Answer from the drawing. Dimensions are ordinates in mm from the lowest x, y and z of the part. Coordinates: 2 decimals unless noted, no trailing zeros. Write each loop counter-clockwise with the first axis right and the second up, starting at its lowest first coordinate (ties: lowest second). Pieces come first, ordered by that corner, then holes. Notation, with made-up numbers: M 63,-11 L 84,-11 A24 cw 84,24 Z; hole C 28.5,87 d7. An arc over 180 degrees is marked long. Put each result on its own line as item: value. Start each with the question number.
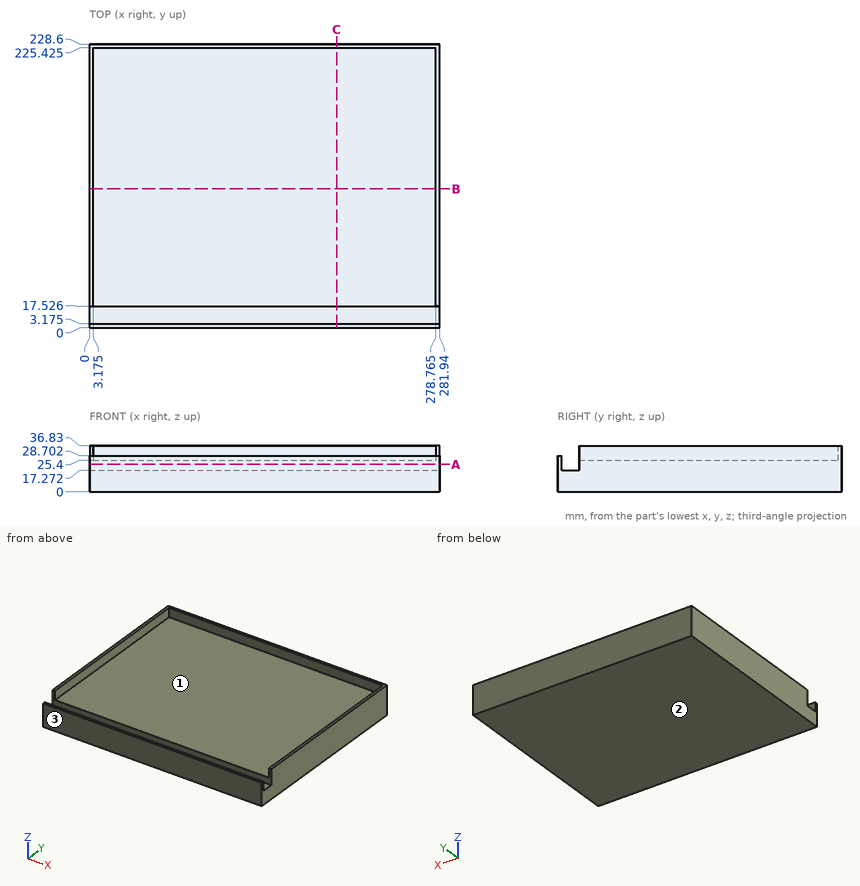
1) A cutting plane is placed at C-C on x = 199. Write down the section's boundary in (y, z) (3 decimals).
2) Determine the mould class of the marked faces 1, 2 and 3 for opening direction Y: +Y half, -Y half, draft (parallel to the pull), parting line (faces both ways), or undercut.
3) Given pin 1 Ø16 at (x, y) = (81.5, 7.5) entering from +Z; pin 2 Ø10 at (x, y) = (57.5, 185.5) entering from +Z; pin 3 Ø3.5 at (x, z) = (150, 33) entering from -Y (3 decimals), each flat-ended and moving along its own axis, determine where each tip first touches the part or whether it passes through.
4) A cutting plane is placed at B-B on y = 112. Write down the section's boundary in (x, z) (3 decimals).
5) Straight lines are drawn through the part: probe 1 along X at (y, z) = (146.5, 27) (3 decimals); probe 2 along Y at (x, z) = (138, 23) (3 decimals); probe 3 along Y at (x, z) = (58, 27) (3 decimals). For each, find the intervals that lie inside material, in ascending order.
6) A cutting plane is placed at A-A on z = 22. Write down the section's boundary in (x, y) (3 decimals), then the cut area to 3 significant figures.
Answers follow:
1. outline: M 0,0 L 228.6,0 L 228.6,36.83 L 225.425,36.83 L 225.425,25.4 L 17.526,25.4 L 17.526,17.272 L 3.175,17.272 L 3.175,28.702 L 0,28.702 Z
2. face 1: undercut
2. face 2: draft
2. face 3: -Y half
3. pin 1: stops at z = 28.7
3. pin 2: stops at z = 25.4
3. pin 3: stops at y = 225.425
4. outline: M 0,0 L 281.94,0 L 281.94,36.83 L 278.765,36.83 L 278.765,25.4 L 3.175,25.4 L 3.175,36.83 L 0,36.83 Z
5. probe 1: x = 0 to 3.175, 278.765 to 281.94
5. probe 2: y = 0 to 3.175, 17.526 to 228.6
5. probe 3: y = 0 to 3.175, 225.425 to 228.6
6. outline: M 0,0 L 281.94,0 L 281.94,3.175 L 0,3.175 Z; M 0,17.526 L 281.94,17.526 L 281.94,228.6 L 0,228.6 Z
6. area: 60,400 mm²
